Geometry check sheet. Reference: the model listing, model coordinates, mm. Coordinates: 2 decimals unless noted, no trailing zeros. Order: outer loops, then holes, each group sorted by start corner. A loop starts at its lowest first (then second) coordinate and runs counter-clockwise, first axis right, second up. Notation, with made-up numbers: (-22, -16.5) - (26, -16.5) arc R17 ccw to (26, 2.5) - close; hole circle Ø2 at (-9, 14.5). An arc over 180 degrees is marked (long way). Use CSV: the item, a comma, the result in double quotes. Start each with the question number.
1) Sectioned sample at C-C, the plane y = 145. Record the cut outline in (x, z), and give its area (3 significant figures).
2) Thickness scan on probe 1 along X at (y, z) = (-53, 3.4); probe 2 along Y at (x, z) = (-152.5, 2.35); probe 3 along X at (y, z) = (175, 2.15). Record the ranges inside material, lowest first. Write a range as [from, to].
3) Depth check by flat-ended pin: P1, Ø3, axis at x = -175, y = 175, coming from the -Z side (3 decimals). Enter the tip coordinate at first touch or a pass-through.
4) Sectioned sample at A-A, the plane y = 35.5. Record the cut outline in (x, z).
5) Sectioned sample at B-B, the plane x = -52. Record the cut outline in (y, z), and give its area (3 significant figures).
6) Sectioned sample at D-D, the plane z = 3. Count the separate pieces of the cut face and the enclosed holes in it, and give its area (3 significant figures).
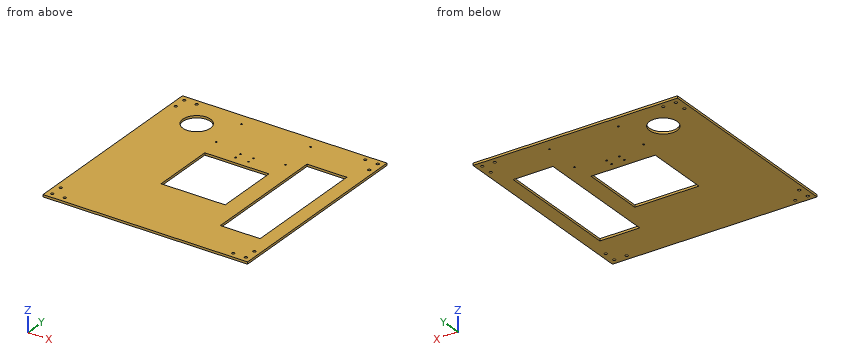
from build123d import *

# Parameters (mm, degrees)
SKETCH_1_W           = 370
SKETCH_1_H           = 370
EXTRUDE_1_DEPTH      = 4
SKETCH_2_R           = 2.5
CUT_EXTRUDE_1_DEPTH  = 262.660084843
SKETCH_6_R           = 1.5
CUT_EXTRUDE_7_DEPTH  = 262.660084843
SKETCH_7_R           = 25
CUT_EXTRUDE_8_DEPTH  = 262.660084843
SKETCH_8_W           = 116
SKETCH_8_H           = 116
CUT_EXTRUDE_9_DEPTH  = 10
SKETCH_11_W          = 72
SKETCH_11_H          = 230
CUT_EXTRUDE_11_DEPTH = 5
SKETCH_12_R          = 1.5
CUT_EXTRUDE_12_DEPTH = 262.660084843


with BuildPart() as part:
    # 草图1 → 凸台-拉伸1 (new body)
    with BuildSketch(Plane.XY):
        Rectangle(SKETCH_1_W, SKETCH_1_H)
    extrude(amount=EXTRUDE_1_DEPTH)

    # 草图2 → 切除-拉伸1 (cut, through all)
    with BuildSketch(Plane.XY.offset(4)):
        with Locations((-175, -175)):
            Circle(SKETCH_2_R)
        with Locations((-152.5, -175)):
            Circle(SKETCH_2_R)
        with Locations((-175, -152.5)):
            Circle(SKETCH_2_R)
        with Locations((-152.5, 175)):
            Circle(SKETCH_2_R)
        with Locations((-175, 152.5)):
            Circle(SKETCH_2_R)
        with Locations((-175, 175)):
            Circle(SKETCH_2_R)
        with Locations((175, 152.5)):
            Circle(SKETCH_2_R)
        with Locations((152.5, 175)):
            Circle(SKETCH_2_R)
        with Locations((175, 175)):
            Circle(SKETCH_2_R)
        with Locations((152.5, -175)):
            Circle(SKETCH_2_R)
        with Locations((175, -152.5)):
            Circle(SKETCH_2_R)
        with Locations((175, -175)):
            Circle(SKETCH_2_R)
    extrude(amount=-CUT_EXTRUDE_1_DEPTH, mode=Mode.SUBTRACT)

    # 草图6 → 切除-拉伸7 (cut, through all)
    with BuildSketch(Plane(origin=(0, 0, 0), x_dir=(-1, 0, 0), z_dir=(0, 0, -1))):
        with Locations((-62.5, 162.249795252)):
            Circle(SKETCH_6_R)
        with Locations((-62.5, 95.249795252)):
            Circle(SKETCH_6_R)
        with Locations((62.5, 95.249795252)):
            Circle(SKETCH_6_R)
        with Locations((62.5, 162.249795252)):
            Circle(SKETCH_6_R)
    extrude(amount=-CUT_EXTRUDE_7_DEPTH, mode=Mode.SUBTRACT)

    # 草图7 → 切除-拉伸8 (cut, through all)
    with BuildSketch(Plane(origin=(0, 0, 0), x_dir=(-1, 0, 0), z_dir=(0, 0, -1))):
        with Locations((118.769854949, 125.631801741)):
            Circle(SKETCH_7_R)
    extrude(amount=-CUT_EXTRUDE_8_DEPTH, mode=Mode.SUBTRACT)

    # 草图8 → 切除-拉伸9 (cut)
    with BuildSketch(Plane(origin=(0, 0, 0), x_dir=(-1, 0, 0), z_dir=(0, 0, -1))):
        Rectangle(SKETCH_8_W, SKETCH_8_H)
    extrude(amount=-CUT_EXTRUDE_9_DEPTH, mode=Mode.SUBTRACT)

    # 草图11 → 切除-拉伸11 (cut)
    with BuildSketch(Plane(origin=(0, 0, 0), x_dir=(-1, 0, 0), z_dir=(0, 0, -1))):
        with Locations((-124, 0)):
            Rectangle(SKETCH_11_W, SKETCH_11_H)
    extrude(amount=-CUT_EXTRUDE_11_DEPTH, mode=Mode.SUBTRACT)

    # 草图12 → 切除-拉伸12 (cut, through all)
    with BuildSketch(Plane(origin=(0, 0, 0), x_dir=(-1, 0, 0), z_dir=(0, 0, -1))):
        with Locations((-11.5, 71.732050808)):
            Circle(SKETCH_12_R)
        with Locations((11.5, 71.732050808)):
            Circle(SKETCH_12_R)
        with Locations((-11.5, 84.732050808)):
            Circle(SKETCH_12_R)
        with Locations((11.5, 84.732050808)):
            Circle(SKETCH_12_R)
    extrude(amount=-CUT_EXTRUDE_12_DEPTH, mode=Mode.SUBTRACT)


solid = part.part
Evaluation:
1,outline,"(-185, 0) - (-134.58, 0) - (-134.58, 4) - (-185, 4) - close; (-102.96, 0) - (185, 0) - (185, 4) - (-102.96, 4) - close"
1,area,"1,350 mm²"
2,probe 1,"[-185, -58], [58, 88], [160, 185]"
2,probe 2,"[-185, -177.5], [-172.5, 172.5], [177.5, 185]"
2,probe 3,"[-185, -177.5], [-172.5, -155], [-150, 150], [155, 172.5], [177.5, 185]"
3,P1,"through"
4,outline,"(-185, 0) - (-58, 0) - (-58, 4) - (-185, 4) - close; (58, 0) - (88, 0) - (88, 4) - (58, 4) - close; (160, 0) - (185, 0) - (185, 4) - (160, 4) - close"
5,outline,"(-185, 0) - (-58, 0) - (-58, 4) - (-185, 4) - close; (58, 0) - (185, 0) - (185, 4) - (58, 4) - close"
5,area,"1,020 mm²"
6,separate pieces,"1"
6,enclosed holes,"23"
6,area,"105,000 mm²"
